```python
from build123d import *

# Parameters (mm, degrees)
BOSS_EXTRUDE1_DEPTH = 76.2
SKETCH2_R           = 15.24
CUT_EXTRUDE1_DEPTH  = 38.1
SKETCH3_R           = 17.78
CUT_EXTRUDE2_DEPTH  = 6.35
CUT_EXTRUDE3_DEPTH  = 12.7
CUT_EXTRUDE4_DEPTH  = 26.4
SKETCH6_W           = 82.55
SKETCH6_H           = 76.2
CUT_EXTRUDE5_DEPTH  = 0.762
BOSS_EXTRUDE2_DEPTH = 7.62
LPATTERN1_COUNT     = 2
LPATTERN1_PITCH     = 26.67


with BuildPart() as part:
    # Sketch1 → Boss-Extrude1 (new body)
    with BuildSketch(Plane(origin=(0, 0, 0), x_dir=(1, 0, 0), z_dir=(0, 1, 0))):
        with BuildLine():
            Line((0, 0), (0, 45.6184))
            ThreePointArc((0, 45.6184), (11.4808, 57.0992), (0, 68.58))
            Line((0, 68.58), (0, 82.55))
            Line((0, 82.55), (25.4, 82.55))
            Line((25.4, 82.55), (25.4, 0))
            Line((25.4, 0), (0, 0))
        make_face()
    extrude(amount=BOSS_EXTRUDE1_DEPTH)

    # Sketch2 → Cut-Extrude1 (cut)
    with BuildSketch(Plane.XZ):
        with Locations((0, -57.0992)):
            Circle(SKETCH2_R)
    extrude(amount=-CUT_EXTRUDE1_DEPTH, mode=Mode.SUBTRACT)

    # Sketch3 → Cut-Extrude2 (cut)
    with BuildSketch(Plane(origin=(0, 16.51, 0), x_dir=(-1, 0, 0), z_dir=(0, -1, 0))):
        with Locations((0, 57.0992)):
            Circle(SKETCH3_R)
    extrude(amount=-CUT_EXTRUDE2_DEPTH, mode=Mode.SUBTRACT)

    # Sketch4 → Cut-Extrude3 (cut)
    with BuildSketch(Plane.ZY):
        with BuildLine():
            Line((-57.0992, 0), (-12.6492, 0))
            Line((-12.6492, 0), (-12.6492, 15.24))
            ThreePointArc((-12.6492, 15.24), (-19.344738982, 31.404461018), (-35.5092, 38.1))
            Line((-35.5092, 38.1), (-57.0992, 38.1))
            Line((-57.0992, 38.1), (-57.0992, 0))
        make_face()
    extrude(amount=-CUT_EXTRUDE3_DEPTH, mode=Mode.SUBTRACT)

    # Sketch5 → Cut-Extrude4 (cut, through all)
    with BuildSketch(Plane(origin=(25.4, 0, 0), x_dir=(0, 0, -1), z_dir=(1, 0, 0))):
        with BuildLine():
            Line((0, 76.2), (31.6484, 76.2))
            Line((31.6484, 76.2), (31.6484, 47.625))
            Line((31.6484, 47.625), (9.525, 47.625))
            ThreePointArc((9.525, 47.625), (2.789807909, 44.835192091), (0, 38.1))
            Line((0, 38.1), (0, 76.2))
        make_face()
    extrude(amount=-CUT_EXTRUDE4_DEPTH, mode=Mode.SUBTRACT)

    # Sketch6 → Cut-Extrude5 (cut)
    with BuildSketch(Plane.ZY):
        with Locations((-41.275, 38.1)):
            Rectangle(SKETCH6_W, SKETCH6_H)
    extrude(amount=-CUT_EXTRUDE5_DEPTH, mode=Mode.SUBTRACT)

    # Sketch9 → Boss-Extrude2 (add)
    with BuildSketch(Plane.XZ):
        with BuildLine():
            Line((0.762, -12.6492), (25.4, -12.6492))
            Line((25.4, -12.6492), (25.4, 19.05))
            Line((25.4, 19.05), (0.762, 19.05))
            Line((0.762, 19.05), (0.762, 11.43))
            ThreePointArc((0.762, 11.43), (4.572, 7.62), (0.762, 3.81))
            Line((0.762, 3.81), (0.762, -12.6492))
        make_face()
        with BuildLine():
            Line((0.762, -72.320138079), (25.4, -72.320138079))
            Line((25.4, -72.320138079), (25.4, -101.6))
            Line((25.4, -101.6), (0.762, -101.6))
            Line((0.762, -101.6), (0.762, -93.98))
            ThreePointArc((0.762, -93.98), (4.572, -90.17), (0.762, -86.36))
            Line((0.762, -86.36), (0.762, -72.320138079))
        make_face()
    boss_extrude2 = extrude(amount=-BOSS_EXTRUDE2_DEPTH)

    # LPattern1: Boss-Extrude2 ×2
    with Locations(*[(0, i * LPATTERN1_PITCH, 0) for i in range(1, LPATTERN1_COUNT)]):
        add(boss_extrude2)


solid = part.part
```
Build history of the part. All positions in model axes, mm. A direction names the side the tool comes from. Round coordinates to 2 decimals unless told otherwise and drop trailing zeros. Order: outer loops, then holes, each group sorted by start corner. A loop starts at its lowest first (then second) coordinate and runs counter-clockwise, first axis right, second up. Notation, with made-up numbers: (58.25, 8.5) - (101.25, 8.5) arc R23 ccw to (101.25, 18.5) - close; hole circle Ø8 at (39.25, 27.25). An arc over 180 degrees is marked (long way). Use a Markdown table: item, result.
1) Tool access for faces 1 (the face through (13, 26.67, -92)), 2 (the face through (10, 38.1, -50)), 3 (the face through (13, 26.67, 10)), 4 (the face through (14, 22.86, -64)), 5 (the face through (4.57, 3.76, 7.7)): list every direction of +Z, -Z, +X, -X, +Y, -Y with a clear straight run to the whole face (end or side of a thin tool).
Recorded:
| item | result |
|---|---|
| face 1 | -Z, +X, -X |
| face 2 | -X, -Y |
| face 3 | +Z, +X, -X |
| face 4 | -X |
| face 5 | -X, +Y, -Y |
2) Saw through at C-C on y = 52. Write the cut outline in (x, z), and give its area (3 significant figures).
Recorded:
| item | result |
|---|---|
| outline | (0.76, -82.55) - (25.4, -82.55) - (25.4, -31.65) - (0.76, -31.65) - (0.76, -45.64) arc R11.48 cw to (0.76, -68.55) - close |
| area | 1,060 mm² |
3) Saw through at D-D on z = -24.5. Write the cut outline in (x, y) (3 decimals).
Recorded:
| item | result |
|---|---|
| outline | (0.762, 35.274) - (12.7, 35.274) - (12.7, 0) - (25.4, 0) - (25.4, 47.625) - (0.762, 47.625) - close |
4) Wall check: L1, parallel to Y at x = 5.75, z = 12; L2, parallel to Y at x = 7, z = -72.5; L3, parallel to Z at x = 2.25, y = 34. Give the ranges that are in metal, low to high.
Recorded:
| item | result |
|---|---|
| L1 | y = 0 to 7.62, 26.67 to 34.29 |
| L2 | y = 0 to 16.51, 22.86 to 76.2 |
| L3 | z = -101.6 to -93.68, -86.66 to -72.17, -22.45 to 4.11, 11.13 to 19.05 |
5) Pull direction Z, two halves, no side cores. Call faces 6 (the face through (16.43, 19.64, -63.9)), 7 (the face through (13, 55, -82.55)), 8 (the face through (0.762, 4, 15)), 9 (the face through (13.253, 44.909, -2.864)): pulls with the +Z half, pulls with the -Z half, needs draft (parallel to the pull), parting line crosses it, or undercut.
Recorded:
| item | result |
|---|---|
| face 6 | undercut |
| face 7 | pulls with the -Z half |
| face 8 | needs draft |
| face 9 | pulls with the +Z half |
6) Flat gauge pins, fed straight in: pin 1 Ø4 at (x, y) = (21.5, 63.5) entering from +Z; pin 2 Ø12 at (x, y) = (4.5, 24.5) entering from -Z; pin 3 Ø1.5 at (x, y) = (9.5, 64) entering from -Z; pin 4 Ø4 at (x, z) = (11.5, -18) entering from +Y (3 decimals). Where does each tip first touch, or does it go through?
Recorded:
| item | result |
|---|---|
| pin 1 | stops at z = -31.65 |
| pin 2 | stops at z = -101.6 |
| pin 3 | stops at z = -82.55 |
| pin 4 | stops at y = 47.625 |
7) Saw through at A-A on z = 7.62. Write the cut outline in (x, y), and give its area (3 significant figures).
Recorded:
| item | result |
|---|---|
| outline | (4.57, 0) - (25.4, 0) - (25.4, 7.62) - (4.57, 7.62) - close; (4.57, 26.67) - (25.4, 26.67) - (25.4, 34.29) - (4.57, 34.29) - close |
| area | 317 mm² |
8) Saw through at B-B on x = 19. Write the cut outline in (y, z) (3 decimals), and give its area (3 significant figures).
Recorded:
| item | result |
|---|---|
| outline | (0, -101.6) - (7.62, -101.6) - (7.62, -82.55) - (26.67, -82.55) - (26.67, -101.6) - (34.29, -101.6) - (34.29, -82.55) - (76.2, -82.55) - (76.2, -31.648) - (47.625, -31.648) - (47.625, -9.525) arc R9.525 ccw to (38.1, 0) - (34.29, 0) - (34.29, 19.05) - (26.67, 19.05) - (26.67, 0) - (7.62, 0) - (7.62, 19.05) - (0, 19.05) - close |
| area | 5,950 mm² |
